from build123d import *

# Parameters (mm, degrees)
SKETCH1_R           = 21
SKETCH1_R_2         = 17.5
BOSS_EXTRUDE1_DEPTH = 4
BOSS_EXTRUDE2_DEPTH = 2.5
SKETCH3_RX          = 2.25
SKETCH3_RY          = 1.6
SKETCH3_RX_2        = 3
SKETCH3_RY_2        = 2
CUT_EXTRUDE1_DEPTH  = 2.5
FILLET1_R           = 3


with BuildPart() as part:
    # Sketch1 → Boss-Extrude1 (new body)
    with BuildSketch(Plane(origin=(0, 0, 0), x_dir=(1, 0, 0), z_dir=(0, 1, 0))):
        with Locations(Location((0, 0, 0), (0, 0, 270))):
            Circle(SKETCH1_R)
        with Locations(Location((0, 0, 0), (0, 0, 270))):
            Circle(SKETCH1_R_2, mode=Mode.SUBTRACT)
    extrude(amount=BOSS_EXTRUDE1_DEPTH)

    # Sketch2 → Boss-Extrude2 (add)
    with BuildSketch(Plane(origin=(0, 4, 0), x_dir=(1, 0, 0), z_dir=(0, 1, 0))):
        Polygon((-20.396078054, 5), (-29.935470069, 2), (-29.935470069, -2), (-20.396078054, -5), align=None)
        Polygon((20.396078054, -5), (20.396078054, 5), (29.935470069, 2), (29.935470069, -2), align=None)
        Polygon((-18, 10.816653826), (-18, 38.816653826), (-4, 38.816653826), (-4, 20.615528128), align=None)
        Polygon((4, 20.615528128), (18, 10.816653826), (18, 38.816653826), (4, 38.816653826), align=None)
    extrude(amount=-BOSS_EXTRUDE2_DEPTH)

    # Sketch3 → Cut-Extrude1 (cut)
    with BuildSketch(Plane(origin=(0, 4, 0), x_dir=(1, 0, 0), z_dir=(0, 1, 0))):
        with Locations(Location((-11, 32.566653826), (0, 0, 90))):
            Ellipse(SKETCH3_RX, SKETCH3_RY)
        with Locations(Location((11, 32.566653826), (0, 0, 90))):
            Ellipse(SKETCH3_RX, SKETCH3_RY)
        with Locations((-23.5, 0)):
            Ellipse(SKETCH3_RX_2, SKETCH3_RY_2)
        with Locations(Location((23.5, 0), (0, 0, 180))):
            Ellipse(SKETCH3_RX_2, SKETCH3_RY_2)
    extrude(amount=-CUT_EXTRUDE1_DEPTH, mode=Mode.SUBTRACT)

    # Fillet1
    # the kernel refuses this fillet: 3 mm, written as the material it adds along each edge
    with BuildSketch(Plane(origin=(-18, 4, -10.816653826), x_dir=(-0.4996806126682358, 0, 0.8662097236371205), z_dir=(0, -1, 0))) as fillet1_piece_1:
        with BuildLine():
            CenterArc((0.804085058, 2.999521034), FILLET1_R, 240.021128247, 28.955024372)
            Line((-0.69495678, 0.400891863), (0, 0))
            ThreePointArc((0, 0), (0.375239694, 0.003352764), (0.750479387, 0))
        make_face()
    extrude(amount=2.5)
    with BuildSketch(Plane(origin=(-4, 4, -20.615528128), x_dir=(0.9932025912341629, 0, -0.11639850843436236), z_dir=(0, -1, 0))) as fillet1_piece_2:
        with BuildLine():
            CenterArc((3.371129229, -2.991569999), FILLET1_R, 94.296279982, 92.388015463)
            Line((0.391521455, -3.340765524), (0, 0))
            ThreePointArc((0, 0), (1.57319364, -0.05901001), (3.14638728, 0))
        make_face()
    extrude(amount=2.5)
    with BuildSketch(Plane(origin=(4, 4, -20.615528128), x_dir=(-0.9932025912341629, 0, -0.11639850843436243), z_dir=(0, -1, 0))) as fillet1_piece_3:
        with BuildLine():
            CenterArc((3.371129229, 2.991569999), FILLET1_R, 173.315704555, 92.388015463)
            Line((0.391521455, 3.340765524), (0, 0))
            ThreePointArc((0, 0), (1.57319364, 0.05901001), (3.14638728, 0))
        make_face()
    extrude(amount=2.5)
    with BuildSketch(Plane(origin=(18, 4, -10.816653826), x_dir=(0.4996806126682291, 0, 0.8662097236371242), z_dir=(0, -1, 0))) as fillet1_piece_4:
        with BuildLine():
            CenterArc((0.804085058, -2.999521034), FILLET1_R, 91.023847381, 28.955024372)
            Line((-0.69495678, -0.400891863), (0, 0))
            ThreePointArc((0, 0), (0.375239694, -0.003352764), (0.750479387, 0))
        make_face()
    extrude(amount=2.5)
    with BuildSketch(Plane(origin=(20.396078054, 4, -5), x_dir=(-0.2729089679529711, 0, -0.9620398615498447), z_dir=(0, -1, 0)), Plane(origin=(-20.396078054, 4, 5), x_dir=(0.2729089679529655, 0, 0.9620398615498462), z_dir=(0, -1, 0))) as fillet1_piece_5:
        with BuildLine():
            CenterArc((1.620157081, 2.998054992), FILLET1_R, 213.295044107, 54.641661907)
            Line((-0.88740746, 1.351203428), (0, 0))
            ThreePointArc((0, 0), (0.756073304, 0.013615053), (1.512146609, 0))
        make_face()
    extrude(amount=2.5)
    with BuildSketch(Plane(origin=(20.396078054, 4, 5), x_dir=(-0.2729089679529669, 0, 0.9620398615498458), z_dir=(0, -1, 0)), Plane(origin=(-20.396078054, 4, -5), x_dir=(0.27290896795296393, 0, -0.9620398615498467), z_dir=(0, -1, 0))) as fillet1_piece_6:
        with BuildLine():
            CenterArc((1.620157081, -2.998054992), FILLET1_R, 92.063293986, 54.641661907)
            Line((-0.88740746, -1.351203428), (0, 0))
            ThreePointArc((0, 0), (0.756073304, -0.013615053), (1.512146609, 0))
        make_face()
    extrude(amount=2.5)
    # the kernel refuses this fillet: 3 mm, written as the material it takes off along each edge
    with BuildSketch(Plane(origin=(-18, 11.5, -38.816653826), x_dir=(0, 0, 1), z_dir=(0, -1, 0)), Plane(origin=(-4, 11.5, -38.816653826), x_dir=(-1, 0, 0), z_dir=(0, -1, 0)), Plane(origin=(4, 11.5, -38.816653826), x_dir=(0, 0, 1), z_dir=(0, -1, 0)), Plane(origin=(18, 11.5, -38.816653826), x_dir=(-1, 0, 0), z_dir=(0, -1, 0))) as fillet1_2_piece_1:
        with BuildLine():
            CenterArc((FILLET1_R, -FILLET1_R), FILLET1_R, 90, 90)
            Line((0, -FILLET1_R), (0, 0))
            Line((0, 0), (FILLET1_R, 0))
        make_face()
    extrude(amount=17.5, mode=Mode.SUBTRACT)
    with BuildSketch(Plane(origin=(29.935470069, 9.503495393, -2), x_dir=(-0.9539392014169457, 0, -0.30000000000000027), z_dir=(0, -1, 0)), Plane(origin=(29.935470069, 9.503495393, 2), x_dir=(0, 0, -1), z_dir=(0, -1, 0)), Plane(origin=(-29.935470069, 9.503495393, 2), x_dir=(0.9539392014169454, 0, 0.3000000000000004), z_dir=(0, -1, 0)), Plane(origin=(-29.935470069, 9.503495393, -2), x_dir=(0, 0, 1), z_dir=(0, -1, 0))) as fillet1_2_piece_2:
        with BuildLine():
            CenterArc((FILLET1_R * 0.733799385705, -FILLET1_R), FILLET1_R, 90, 72.542396876)
            Line((-FILLET1_R * 0.220139815712, -FILLET1_R * 0.7), (0, 0))
            Line((0, 0), (FILLET1_R * 0.733799385705, 0))
        make_face()
    extrude(amount=13.506990786, mode=Mode.SUBTRACT)


solid = part.part
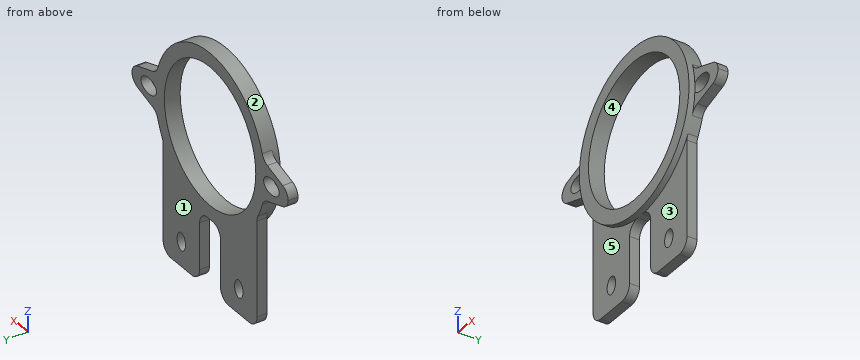
CAD build for the part. Positions are in the model's coordinates, mm. Face numbers are marked on the shaded views. A direction names the side the tool comes from. Round coordinates to 2 decimals unless told otherwise and drop trailing zeros. Order: outer loops, then holes, each group sorted by start corner. A loop starts at its lowest first (then second) coordinate and runs counter-clockwise, first axis right, second up. Notation, with made-up numbers: (-24, 68.25) -> (-14, 68.25) arc R13 cw to (-14, 86.25) -> close; hole circle Ø1 at (-2, 10.25). An arc over 180 degrees is marked (long way). Write each question's results on one line, items separated by ' | '.
1. Cut at B-B (z = -22.5). Give the cut face in (x, y).
Findings below:
outline: (-18, 1.5) -> (-3.61, 1.5) -> (-3.61, 4) -> (-18, 4) -> close; (3.61, 1.5) -> (18, 1.5) -> (18, 4) -> (3.61, 4) -> close
2. Cut at C-C (y = 0.9). Give the cut face in (x, z), plus the area to 3 significant figures.
Findings below:
outline: circle Ø42 at (0, 0); hole circle Ø35 at (0, 0) | area: 423 mm²
3. 3-axis set-ups, long thin cutter, end or side, ignore diameter. For the marked faces 1, 2 and 3: which of +Z, -Z, +X, -X, +Y, -Y reach the whole face in a straight line?
Findings below:
face 1: +Z, -Z, +X, -X, +Y | face 2: -Y | face 3: -Z, +X, -Y
4. Flat gauge pins, fed straight in: P1, Ø3, axis at x = -20, z = 0, coming from the -Y side; P2, Ø5, axis at x = 27.5, z = 1.5, coming from the -Y side; P3, Ø0.8, axis at y = 2.5, z = -31, coming from the +X side; P4, Ø1.2, axis at y = 2.5, z = -32.5, coming from the -X side. Where does each tip first touch, or does it go through?
Findings below:
P1: stops at y = 0 | P2: stops at y = 1.5 | P3: stops at x = 18 | P4: stops at x = -18
5. Wall check: line 1 along X through (y, z) = (1.4, 0); line 2 along X through (y, z) = (3.45, -31.5); line 3 along X through (y, z) = (2, -34). Give the ranges that are in metal, low to high. Write a range as [from, to].
Findings below:
line 1: x = [-21, -17.5], [17.5, 21] | line 2: x = [-18, -12.41], [-9.59, -4], [4, 9.59], [12.41, 18] | line 3: x = [-18, -12.23], [-9.77, -4], [4, 9.77], [12.23, 18]
6. Cut at A-A (x = 0). Give the cut face in (y, z).
Findings below:
outline: (0, -21) -> (4, -21) -> (4, -17.5) -> (0, -17.5) -> close; (0, 17.5) -> (4, 17.5) -> (4, 21) -> (0, 21) -> close
7. Pull direction X, two halves, no side cores. Call the marked faces 4 and 5: pulls with the +X half, pulls with the -X half, needs draft (parallel to the pull), parting line crosses it, or undercut.
Findings below:
face 4: undercut | face 5: needs draft
